from build123d import *

# Parameters (mm, degrees)
BOSS_EXTRUDE1_DEPTH = 5
SKETCH2_R           = 4.01
CUT_EXTRUDE1_DEPTH  = 10


with BuildPart() as part:
    # Sketch1 → Boss-Extrude1 (new body)
    with BuildSketch(Plane.XY):
        with BuildLine():
            Line((90, 10), (0, 10))
            ThreePointArc((0, 10), (-10, 0), (0, -10))
            Line((0, -10), (90, -10))
            ThreePointArc((90, -10), (100, 0), (90, 10))
        make_face()
    extrude(amount=BOSS_EXTRUDE1_DEPTH)

    # Sketch2 → Cut-Extrude1 (cut)
    with BuildSketch(Plane.XY.offset(5)):
        Circle(SKETCH2_R)
        with Locations((90, 0)):
            Circle(SKETCH2_R)
    extrude(amount=-CUT_EXTRUDE1_DEPTH, mode=Mode.SUBTRACT)


solid = part.part
CAD build for the part. Positions are in the model's coordinates, mm. Give positions to 0.01 mm unless a question says otherwise; leave off trailing zeros. Order: outer loops, then holes, each group sorted by start corner. A loop starts at its lowest first (then second) coordinate and runs counter-clockwise, first axis right, second up. Notation, with made-up numbers: (-6.5, -18) - (38.5, -18) arc R21 ccw to (38.5, 7) - close; hole circle Ø9 at (26.5, 63). An arc over 180 degrees is marked (long way). Answer in a Markdown table with one row per item.
1. Saw through at B-B, the plane z = 2.05. Give the cut face in (x, y), plus the area to 3 significant figures.
Data:
| item | result |
|---|---|
| outline | (0, -10) - (90, -10) arc R10 ccw to (90, 10) - (0, 10) arc R10 ccw to start; hole circle Ø8.02 at (0, 0); hole circle Ø8.02 at (90, 0) |
| area | 2,010 mm² |
2. Pull direction Y, two halves, no side cores. Call faces 1 (the cylindrical face through (100, 0, 2)), 2 (the cylindrical face through (-0.869, -3.915, 2.535)), 3 (the flat face through (46, 10, 2)): pulls with the +Y half, pulls with the -Y half, needs draft (parallel to the pull), parting line crosses it, or undercut.
Data:
| item | result |
|---|---|
| face 1 | parting line crosses it |
| face 2 | undercut |
| face 3 | pulls with the +Y half |
3. Probe probe 1 along Y at (x, z) = (0, 3.45); probe 2 along X at (y, z) = (-2.25, 3.7); probe 3 along X at (y, z) = (0.75, 3.4). List the from-to ranges inside material, lowest first. Write a range as [from, to].
Data:
| item | result |
|---|---|
| probe 1 | y = [-10, -4.01], [4.01, 10] |
| probe 2 | x = [-9.74, -3.32], [3.32, 86.68], [93.32, 99.74] |
| probe 3 | x = [-9.97, -3.94], [3.94, 86.06], [93.94, 99.97] |
4. Saw through at A-A, the plane y = 0. Give the cut face in (x, z), plus the area to 3 significant figures.
Data:
| item | result |
|---|---|
| outline | (-10, 0) - (-4.01, 0) - (-4.01, 5) - (-10, 5) - close; (4.01, 0) - (85.99, 0) - (85.99, 5) - (4.01, 5) - close; (94.01, 0) - (100, 0) - (100, 5) - (94.01, 5) - close |
| area | 470 mm² |
5. Saw through at C-C, the plane y = -6. Give the cut face in (x, z), plus the area to 3 significant figures.
Data:
| item | result |
|---|---|
| outline | (-8, 0) - (98, 0) - (98, 5) - (-8, 5) - close |
| area | 530 mm² |
